```python
from build123d import *

# Parameters (mm, degrees)
SKETCH1_W            = 230
SKETCH1_H            = 200
BOSS_EXTRUDE1_DEPTH  = 5
SKETCH2_R            = 15
SKETCH2_R_2          = 14
SKETCH2_R_3          = 10
SKETCH2_R_4          = 18.5
SKETCH2_R_5          = 3
CUT_EXTRUDE1_DEPTH   = 305.836021494
M4_CLEARANCE_HOLE1_D = 4.8
SKETCH5_W            = 20
SKETCH5_H            = 5
CUT_EXTRUDE2_DEPTH   = 305.836021494
SKETCH8_W            = 230
SKETCH8_H            = 89.8
CUT_EXTRUDE4_DEPTH   = 305.836021494
SKETCH16_W           = 120
SKETCH16_H           = 1.1
BOSS_EXTRUDE2_DEPTH  = 5
M8_CLEARANCE_HOLE1_D = 9
CUT_EXTRUDE7_DEPTH   = 306.558848669
M5_CLEARANCE_HOLE2_D = 5.5
FILLET3_R            = 30
SKETCH22_W           = 97.742742711
SKETCH22_H           = 151.745417032
CUT_EXTRUDE8_DEPTH   = 281.162827656
SKETCH23_R           = 5
CUT_EXTRUDE9_DEPTH   = 2.5
FILLET4_R            = 5


with BuildPart() as part:
    # Sketch1 → Boss-Extrude1 (new body)
    with BuildSketch(Plane(origin=(0, 0, 0), x_dir=(1, 0, 0), z_dir=(0, 1, 0))):
        with Locations((115, 100)):
            Rectangle(SKETCH1_W, SKETCH1_H)
    extrude(amount=BOSS_EXTRUDE1_DEPTH)

    # Sketch2 → Cut-Extrude1 (cut, through all)
    with BuildSketch(Plane(origin=(0, 5, 0), x_dir=(1, 0, 0), z_dir=(0, 1, 0))):
        with Locations(Location((50, 60, 0), (0, 0, 270))):
            Circle(SKETCH2_R)
        with Locations(Location((168.717100706, 42.5, 0), (0, 0, 270))):
            Circle(SKETCH2_R_2)
        with Locations(Location((169.895788083, 150, 0), (0, 0, 90))):
            Circle(SKETCH2_R_3)
        with Locations(Location((50, 145, 0), (0, 0, 90))):
            Circle(SKETCH2_R_4)
        with Locations(Location((89.548596028, 156.65798234, 0), (0, 0, 270))):
            Circle(SKETCH2_R_5)
        with BuildLine():
            Line((104.360743639, 72.202850118), (98.527410306, 32.630483216))
            ThreePointArc((98.527410306, 32.630483216), (96.257125294, 30.943531537), (94.570173616, 33.213816549))
            Line((94.570173616, 33.213816549), (100.403506949, 72.786183451))
            ThreePointArc((100.403506949, 72.786183451), (102.673791961, 74.473135129), (104.360743639, 72.202850118))
        make_face()
        with BuildLine():
            Line((94.004324063, 121.813377483), (93.17099073, 141.79600883))
            ThreePointArc((93.17099073, 141.79600883), (90.048596028, 144.668403532), (87.176201326, 141.54600883))
            Line((87.176201326, 141.54600883), (88.009534659, 121.563377483))
            ThreePointArc((88.009534659, 121.563377483), (91.131929361, 118.690982781), (94.004324063, 121.813377483))
        make_face()
    extrude(amount=-CUT_EXTRUDE1_DEPTH, mode=Mode.SUBTRACT)

    # M4 Clearance Hole1 (through all)
    with Locations(Plane(origin=(0, 5, 0), x_dir=(1, 0, 0), z_dir=(0, 1, 0))):
        with Locations((50, 120), (50, 32.5), (168.717100706, 61), (168.717100706, 24), (187.217100706, 42.5), (150.217100706, 42.5), (50, 170)):
            Hole(M4_CLEARANCE_HOLE1_D / 2)

    # Sketch5 → Cut-Extrude2 (cut, through all)
    with BuildSketch(Plane(origin=(0, 5, 0), x_dir=(1, 0, 0), z_dir=(0, 1, 0))):
        with Locations((30, 7.5)):
            Rectangle(SKETCH5_W, SKETCH5_H)
        with Locations((70, 7.5)):
            Rectangle(SKETCH5_W, SKETCH5_H)
        with Locations((110, 7.5)):
            Rectangle(SKETCH5_W, SKETCH5_H)
        with Locations((150, 7.5)):
            Rectangle(SKETCH5_W, SKETCH5_H)
        with Locations((190, 7.5)):
            Rectangle(SKETCH5_W, SKETCH5_H)
    extrude(amount=-CUT_EXTRUDE2_DEPTH, mode=Mode.SUBTRACT)

    # Sketch8 → Cut-Extrude4 (cut, through all)
    with BuildSketch(Plane(origin=(0, 5, 0), x_dir=(1, 0, 0), z_dir=(0, 1, 0))):
        with Locations((115, 44.9)):
            Rectangle(SKETCH8_W, SKETCH8_H)
    extrude(amount=-CUT_EXTRUDE4_DEPTH, mode=Mode.SUBTRACT)

    # Sketch16 → Boss-Extrude2 (add)
    with BuildSketch(Plane(origin=(0, 5, 0), x_dir=(1, 0, 0), z_dir=(0, 1, 0))):
        with Locations((60, 200.55)):
            Rectangle(SKETCH16_W, SKETCH16_H)
    extrude(amount=-BOSS_EXTRUDE2_DEPTH)

    # M8 Clearance Hole1 (through all)
    with Locations(Plane(origin=(0, 5, 0), x_dir=(1, 0, 0), z_dir=(0, 1, 0))):
        with Locations((15, 185.45), (15, 105.45), (105, 105.45), (105, 185.45)):
            Hole(M8_CLEARANCE_HOLE1_D / 2)

    # Sketch18 → Cut-Extrude7 (cut, through all)
    with BuildSketch(Plane(origin=(0, 5, 0), x_dir=(1, 0, 0), z_dir=(0, 1, 0))):
        Polygon((120, 225.92357398), (254.211620271, 225.92357398), (254.211620271, 61.332744885), (120, 61.332744885), (120, 110.45), (195, 110.45), (195, 180.45), (120, 180.45), align=None)
    extrude(amount=-CUT_EXTRUDE7_DEPTH, mode=Mode.SUBTRACT)

    # M5 Clearance Hole2 (through all)
    with Locations(Plane(origin=(0, 5, 0), x_dir=(1, 0, 0), z_dir=(0, 1, 0))):
        with Locations((124.9, 160.45), (124.9, 130.45)):
            Hole(M5_CLEARANCE_HOLE2_D / 2)

    # Fillet3
    fillet3_edges = [part.edges().sort_by_distance(p)[0] for p in [
        (195, 2.5, -110.45),
        (195, 2.5, -180.45),
    ]]
    fillet(fillet3_edges, radius=FILLET3_R)

    # Sketch22 → Cut-Extrude8 (cut, through all)
    with BuildSketch(Plane(origin=(0, 5, 0), x_dir=(1, 0, 0), z_dir=(0, 1, 0))):
        with Locations((183.771371356, 144.05197651)):
            Rectangle(SKETCH22_W, SKETCH22_H)
    extrude(amount=-CUT_EXTRUDE8_DEPTH, mode=Mode.SUBTRACT)

    # Sketch23 → Cut-Extrude9 (cut)
    with BuildSketch(Plane.XZ):
        with Locations(Location((89.548596028, -156.65798234, 0), (0, 0, 270))):
            Circle(SKETCH23_R)
        with BuildLine():
            Line((95.169253864, -141.879342163), (96.002587198, -121.896710816))
            ThreePointArc((96.002587198, -121.896710816), (91.215262694, -116.692719646), (86.011271524, -121.480044149))
            Line((86.011271524, -121.480044149), (85.177938191, -141.462675497))
            ThreePointArc((85.177938191, -141.462675497), (89.965262694, -146.666666667), (95.169253864, -141.879342163))
        make_face()
    extrude(amount=-CUT_EXTRUDE9_DEPTH, mode=Mode.SUBTRACT)

    # Fillet4
    fillet4_edges = [part.edges().sort_by_distance(p)[0] for p in [
        (0, 2.5, -89.8),
        (120, 2.5, -201.1),
        (0, 2.5, -201.1),
        (120, 2.5, -89.8),
        (120, 2.5, -180.45),
        (120, 2.5, -110.45),
        (134.9, 2.5, -180.45),
        (134.9, 2.5, -110.45),
    ]]
    fillet(fillet4_edges, radius=FILLET4_R)


solid = part.part
```
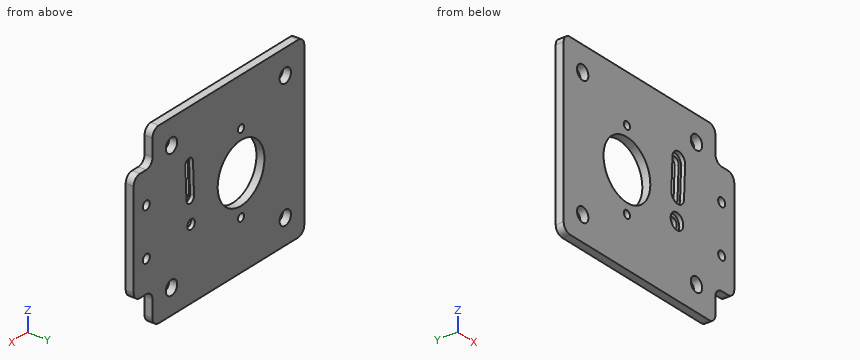
For this review, take the finished solid that the model builds, in its own axes (mm). Give positions to 0.01 mm unless a question says otherwise; leave off trailing zeros. Write each loop counter-clockwise with the first axis right and the second up, starting at its lowest first coordinate (ties: lowest second). Pieces come first, ordered by that corner, then holes. Notation, with made-up numbers: M 63.25,86.5 L 77.25,86.5 A12 cw 77.25,102.5 Z; hole C -35,-36.5 d9. An arc over 180 degrees is marked long. Answer as a JSON object with one key per item and string values. Group by question number.
Item 1: Consider section B-B on x = 50. Write out the cut boundary in (y, z), plus the area to 4 significant figures.
Item 2: For pin 1 Ø11.5 at (x, z) = (105, -105.45) entering from -Y; pin 2 Ø5 at (x, z) = (124.9, -130.45) entering from -Y; pin 3 Ø8.5 at (x, z) = (90.5, -130) entering from -Y; pin 4 Ø1.5 at (y, z) = (1.5, -99.5) entering from +X, all flat-tipped, find the tip position at first contact; note any pin that passes through.
Item 3: Consider section A-A on z = -170. Write out the cut boundary in (x, y).
Item 4: Consider section D-D on y = 3.7. Count the separate pieces of the cut face and the enclosed holes in it, plus the area to 3 significant figures.
Item 5: Consider section C-C on x = 15. Write out the cut boundary in (y, z).
Item 6: For probe 1 along Z at (x, y) = (105, 1.7); probe 2 along X at (y, z) = (1.3, -185); probe 3 along X at (y, z) = (2.05, -120), list the stretches that pass through material, from the lowest coordinate up. Write a range as [from, to].
Check result:
{
 "1": {"outline": "M 0,-201.1 L 5,-201.1 L 5,-172.4 L 0,-172.4 Z; M 0,-167.6 L 5,-167.6 L 5,-163.5 L 0,-163.5 Z; M 0,-126.5 L 5,-126.5 L 5,-122.4 L 0,-122.4 Z; M 0,-117.6 L 5,-117.6 L 5,-89.8 L 0,-89.8 Z", "area": "323.5 mm^2"},
 "2": {"pin 1": "stops at y = 0", "pin 2": "passes through", "pin 3": "stops at y = 2.5", "pin 4": "stops at x = 120"},
 "3": {"outline": "M 0,0 L 47.6,0 L 47.6,5 L 0,5 Z; M 52.4,0 L 134.9,0 L 134.9,5 L 52.4,5 Z"},
 "4": {"separate pieces": "1", "enclosed holes": "11", "area": "12,800 mm^2"},
 "5": {"outline": "M 0,-201.1 L 5,-201.1 L 5,-189.95 L 0,-189.95 Z; M 0,-180.95 L 5,-180.95 L 5,-109.95 L 0,-109.95 Z; M 0,-100.95 L 5,-100.95 L 5,-89.8 L 0,-89.8 Z"},
 "6": {"probe 1": "z = [-201.1, -189.95], [-180.95, -109.95], [-100.95, -89.8]", "probe 2": "x = [0, 10.52], [19.48, 100.52], [109.48, 120.02]", "probe 3": "x = [0, 47.6], [52.4, 86.3], [95.71, 134.9]"}
}
